Study the drawing (mm; zero at the part's minimum x, y, z) and answer. Round coordinates to 2 decimals unless told otherwise and drop trailing zeros. Write each loop counter-clockwise with the first axis right and the second up, starting at its lowest first coordinate (ties: lowest second). Pieces come first, ordered by that corner, then holes.
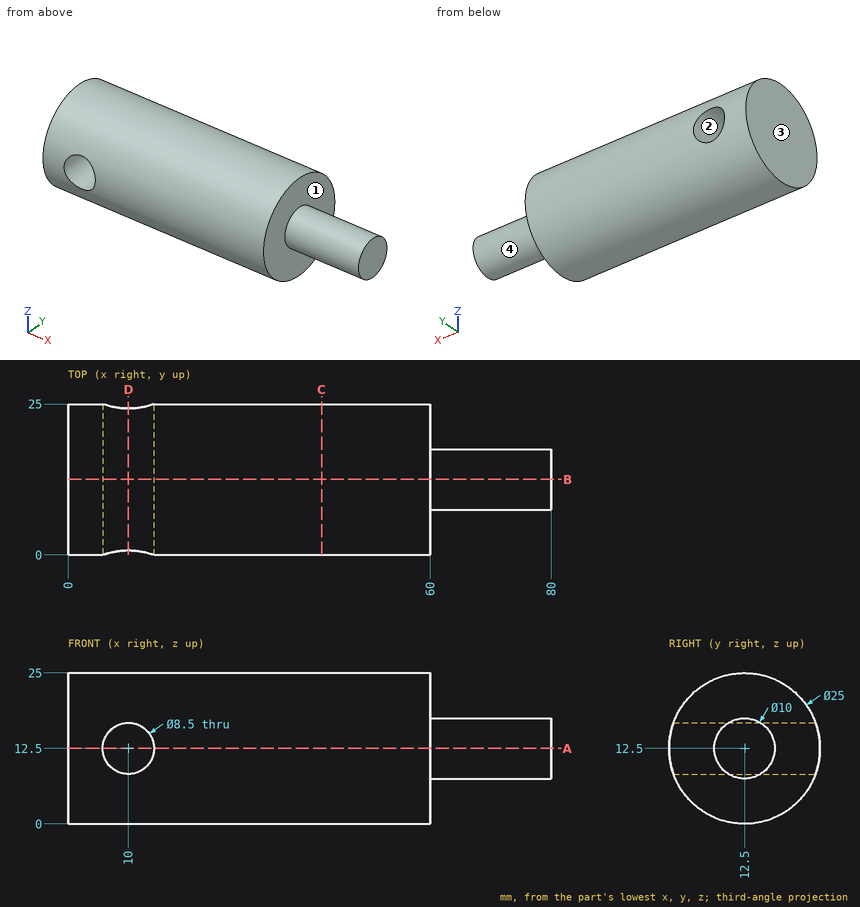
Q1. Find section C-C (x = 42). Determine the outline of the cut face in (y, z), plus the area to 3 significant figures.
Q2. Find section D-D (x = 10). Determine the outline of the cut face in (y, z).
Q3. Find section A-A (z = 12.5). Determine the outline of the cut face in (x, y).
Q4. Given pin 1 (7 mm diameter, centred on x = 10, z = 12.5, fed in from -Y) (3 decimals); pin 2 (2 mm diameter, centred on x = 45.5, z = 5.5, fed in from +Y); pin 3 (7.5 mm diameter, centred on y = 10.5, z = 6.5, fed in from +X); pin 4 (1 mm diameter, centred on y = 20, z = 9.5, fed in from +X), each flat-ended and moving along its own axis, determine where each tip first touches the part or whether it passes through.
Q5. Find section B-B (y = 12.5). Determine the outline of the cut face in (x, z).
Q6. Find the intervals of material crossed by L1, parallel to Z at x = 10, y = 12.75; L2, parallel to Z at x = 10, y = 6; L3, parallel to X at y = 12.5, z = 23.5, in increasing order.
Q7. The mould has two halves that part along X. Classify the marked faces 1, 2, 3 and 4: +X half, -X half, draft (parallel to the pull), parting line (faces both ways), or undercut.
Report:
1. outline: circle Ø25 at (12.5, 12.5)
1. area: 491 mm2
2. outline: (0.74, 8.25) arc R12.5 ccw to (24.26, 8.25) - close; (0.74, 16.75) - (24.26, 16.75) arc R12.5 ccw to start
3. outline: (0, 0) - (5.75, 0) - (5.75, 25) - (0, 25) - close; (14.25, 0) - (60, 0) - (60, 7.5) - (80, 7.5) - (80, 17.5) - (60, 17.5) - (60, 25) - (14.25, 25) - close
4. pin 1: passes through
4. pin 2: stops at y = 23.47
4. pin 3: stops at x = 80
4. pin 4: stops at x = 60
5. outline: (0, 0) - (60, 0) - (60, 7.5) - (80, 7.5) - (80, 17.5) - (60, 17.5) - (60, 25) - (0, 25) - close; hole circle Ø8.5 at (10, 12.5)
6. L1: z = 0 to 8.25, 16.75 to 25
6. L2: z = 1.82 to 8.25, 16.75 to 23.18
6. L3: x = 0 to 60
7. face 1: +X half
7. face 2: undercut
7. face 3: -X half
7. face 4: draft
